from build123d import *

# Parameters (mm, degrees)
BOSS_EXTRUDE1_DEPTH = 6.35
SKETCH2_W           = 177.8
SKETCH2_H           = 460.375
CUT_EXTRUDE1_DEPTH  = 7.35
SKETCH3_W           = 2150.099514553
SKETCH3_H           = 1524
CUT_EXTRUDE2_DEPTH  = 7.35


with BuildPart() as part:
    # Sketch1 → Boss-Extrude1 (new body)
    with BuildSketch(Plane(origin=(0, 0, 0), x_dir=(1, 0, 0), z_dir=(0, 1, 0))):
        Polygon((-914.4, 0), (914.4, 0), (914.4, 3048), (-914.4, 3048), (-1438.899514553, 3048), (-1438.899514553, 0), align=None)
    extrude(amount=BOSS_EXTRUDE1_DEPTH)

    # Sketch2 → Cut-Extrude1 (cut, through all)
    with BuildSketch(Plane(origin=(0, 6.35, 0), x_dir=(1, 0, 0), z_dir=(0, 1, 0))):
        Polygon((914.4, 0), (533.4, 0), (533.4, 460.375), (711.2, 460.375), (711.2, 2587.625), (533.4, 2587.625), (533.4, 3048), (914.4, 3048), (914.4, 2587.625), (914.4, 460.375), align=None)
        with Locations((-1349.999514553, 230.1875)):
            Rectangle(SKETCH2_W, SKETCH2_H)
        with Locations((-1349.999514553, 2817.8125)):
            Rectangle(SKETCH2_W, SKETCH2_H)
    extrude(amount=-CUT_EXTRUDE1_DEPTH, mode=Mode.SUBTRACT)

    # Sketch3 → Cut-Extrude2 (cut, through all)
    with BuildSketch(Plane(origin=(0, 6.35, 0), x_dir=(1, 0, 0), z_dir=(0, 1, 0))):
        with Locations((-363.849757276, 2286)):
            Rectangle(SKETCH3_W, SKETCH3_H)
    extrude(amount=-CUT_EXTRUDE2_DEPTH, mode=Mode.SUBTRACT)


solid = part.part
Verification items for the finished model (mm, model axes). Coordinates: 2 decimals unless noted, no trailing zeros. Order: outer loops, then holes, each group sorted by start corner. A loop starts at its lowest first (then second) coordinate and runs counter-clockwise, first axis right, second up.
1. Scan lines: line 1 (X direction, y = 0.75, z = -215); line 2 (Z direction, x = 592.5, y = 5.5) (3 decimals). Record each from-to range of solid material in increasing order.
Results found:
line 1: x = -1261.1 to 533.4
line 2: z = -1524 to -460.375
2. Go/stop test with flat-tipped pins: pin 1 Ø1.9 at (x, y) = (-1336.5, 2) entering from +Z (3 decimals); pin 2 Ø3 at (y, z) = (3, -142.5) entering from -X. Record where each tip stops, or that it passes through.
Results found:
pin 1: stops at z = -460.375
pin 2: stops at x = -1261.1
3. Sectioned sample at B-B, the plane z = -316. Record the cut outline in (x, y), and give its area (3 significant figures).
Results found:
outline: (-1261.1, 0) - (533.4, 0) - (533.4, 6.35) - (-1261.1, 6.35) - close
area: 11,400 mm2
4. Sectioned sample at A-A, the plane y = 2. Record the cut outline in (x, z) (3 decimals), and give its area (3 significant figures).
Results found:
outline: (-1438.9, -1524) - (711.2, -1524) - (711.2, -460.375) - (533.4, -460.375) - (533.4, 0) - (-1261.1, 0) - (-1261.1, -460.375) - (-1438.9, -460.375) - close
area: 3,110,000 mm2
